Autodesk Inventor part; units mm, degrees
ref_plane "YZ Plane" through (0, 0, 0) normal (1, 0, 0) x (0, 1, 0)
ref_plane "XZ Plane" through (0, 0, 0) normal (0, 1, 0) x (-1, 0, 0)
ref_plane "XY Plane" through (0, 0, 0) normal (0, 0, 1) x (1, 0, 0)
sketch "Sketch1" plane through (0, 0, 0) normal (0, 0, 1) x (1, 0, 0)
  circle A0 centre (0, 0) radius 2.5
  dimension "d0" = 5
sketch "Sketch2" plane through (0, 0, 0) normal (1, 0, 0) x (0, 1, 0)
  line L0 (0, 0) -> (0, -15.5)
  line L1 (7.5, -23) -> (32.5, -23)
  arc A0 (0, -15.5) -> (7.5, -23) centre (7.5, -15.5) ccw
  point P0 (0, -23)
  dimension "d1" = 23
  dimension "d2" = 7.5
  dimension "d3" = 25
sweep "Sweep1" add profiles "Sketch1" path "Sketch2"
sketch "Sketch3" plane through (0, 0, 0) normal (0, 0, 1) x (1, 0, 0)
  circle A0 centre (0, 0) radius 3
  dimension "d6" = 6
extrude "Extrusion1" add sketch "Sketch3" along normal mid plane 12
shell "Shell1" thickness 0.5 removed faces 2 at (-0.5351, 1.0949, 6) at (-0.2146, 32.5, -22.3381)
properties part number "161" material "Iron, Cast"
Verification items for the finished model (mm, model axes). A direction names the side the tool comes from. Coordinates: 2 decimals unless noted, no trailing zeros. Write each loop counter-clockwise with the first axis right and the second up, starting at its lowest first coordinate (ties: lowest second). Pieces come first, ordered by that corner, then holes. Notation, with made-up numbers: M 73,48.5 L 90,48.5 A18 cw 90,53.5 Z; hole C 28.5,57 d3. An arc over 180 degrees is marked long. Use CSV: the item, a comma, the result in double quotes.
Q1. Section check A-A, the plane x = 0. Enter the section's corners in (y, z), and give its area (3 significant figures).
Computed values:
outline,"M -3,-6 L -2.5,-6 L -2.5,-15.5 A10 ccw 7.5,-25.5 L 32.5,-25.5 L 32.5,-25 L 7.5,-25 A9.5 cw -2,-15.5 L -2,-5.5 L -2.5,-5.5 L -2.5,6 L -3,6 Z; M 2,-15.5 A5.5 ccw 7.5,-21 L 32.5,-21 L 32.5,-20.5 L 7.5,-20.5 A5 cw 2.5,-15.5 L 2.5,-6 L 3,-6 L 3,6 L 2.5,6 L 2.5,-5.5 L 2,-5.5 Z"
area,"58.8 mm²"
Q2. Go/stop test with flat-tipped pins: P1, Ø3.5, axis at x = 0, z = -23, coming from the -Y side; P2, Ø3, axis at x = 0, y = 0, coming from the -Z side; P3, Ø1.5, axis at x = -2, y = 12.5, coming from the -Z side. Record where each tip stops, or that it passes through.
Computed values:
P1,"y = -0.68"
P2,"z = -23.5"
P3,"z = -25.17"
Q3. Mould release check, pull along Y, two halves, no side actions. Record for faces 1 (the flat face through (2, 32.5, -22)), 2 (the cylindrical face through (0, 2, -11)), 3 (the cylindrical face through (-3, 0, 0)): pulls with the +Y half, pulls with the -Y half, needs draft (parallel to the pull), parting line crosses it, or undercut.
Computed values:
face 1,"pulls with the +Y half"
face 2,"undercut"
face 3,"parting line crosses it"
Q4. Section check C-C, the plane y = 20.5. Enter the section's corners in (x, z), and give its area (3 significant figures).
Computed values:
outline,"C 0,-23 d5; hole C 0,-23 d4"
area,"7.07 mm²"
Q5. Set-up check for faces 4 (the cylindrical face through (-0.54, 2.44, -10.82)), 5 (the flat face through (-2, 2, 6)), 6 (the cylindrical face through (0.923, 20.175, -21.226)), 7 (the flat face through (-1, 2, -5.5)): record each of +Z, -Z, +X, -X, +Y, -Y from which the full face is reachable in a straight line by a thin tool's end or side.
Computed values:
face 4,"none"
face 5,"+Z, +X, -X, +Y, -Y"
face 6,"+Y"
face 7,"+Z"
Q6. Section check B-B, the plane z = -14. Enter the section's corners in (x, y).
Computed values:
outline,"C 0,0 d5; hole C 0,0 d4"
Q7. Thickness scan on line 1 along Y through (x, z) = (0, 1.75); line 2 along Y through (x, z) = (0, -13); line 3 along Z through (x, y) = (0.1, 17.5). Record the ranges inside material, lowest first. Write a range as [from, to].
Computed values:
line 1,"[-3, -2.5], [2.5, 3]"
line 2,"[-2.5, -2], [2, 2.5]"
line 3,"[-25.5, -25], [-21, -20.5]"
